The model under review builds one solid part; all positions refer to its coordinate system, in mm. A direction names the side the tool comes from. Round coordinates to 2 decimals unless told otherwise and drop trailing zeros. Order: outer loops, then holes, each group sorted by start corner. A loop starts at its lowest first (then second) coordinate and runs counter-clockwise, first axis right, second up. Notation, with made-up numbers: M 46.5,-16.5 L 102.5,-16.5 A25 cw 102.5,4.5 Z; hole C -39,36.5 d5. An arc over 180 degrees is marked long. Answer as a JSON object with one key per item and string values. Group by question number.
1) Consider section C-C, the plane x = 13. Write out the cut boundary in (y, z), then the cut area to 3 significant figures.
2) Insertion check: pin 1 Ø2 at (x, z) = (18.5, 14.5) entering from -Y; pin 2 Ø10 at (x, z) = (-16, 21) entering from +Y. Each pin has a flat end and moves straight along its axis. Give the tip position at first contact, or say it passes through.
3) Consider section A-A, the plane z = 0. Write out the cut boundary in (x, y), then the cut area to 3 significant figures.
4) Consider section B-B, the plane x = 0. Write out the cut boundary in (y, z).
5) To check wall thickness, follow line 1 (X direction, y = 33.5, z = 0); line 2 (Y direction, x = 17, z = 8); line 3 (Y direction, x = -23, z = -7). State the ranges of each line that lie inside material, in increasing order.
6) Consider section D-D, the plane y = 32.75. Write out the cut boundary in (x, z), then the cut area to 3 significant figures.
7) For faces 1 (the cylindrical face through (20.013, 37.121, 4.444)), 2 (the cylindrical face through (0, 35, 22)), 3 (the flat face through (0, 34.1, -5)), list the 3-axis set-ups (+Z, -Z, +X, -X, +Y, -Y) from which the entire face can be reached by the end or side of a thin tool; tool diameter is ignored.
8) The part is to be moulded in two halves that separate along Z. For faces 4 (the flat face through (14, 35.6, -16)), 5 (the cylindrical face through (7.46, 34.84, -22.37)), 6 (the cylindrical face through (-26.274, 33.135, 3.45)), say which applies: +Z half, -Z half, draft (parallel to the pull), parting line (faces both ways), or undercut.
```python
from build123d import *

# Parameters (mm, degrees)
SKETCH_3_W          = 2.645592797
SKETCH_3_H          = 5.492550126
CUT_EXTRUDE_START   = -20
CUT_EXTRUDE_2_DEPTH = 20
CUT_EXTRUDE_START_2 = -10
CUT_EXTRUDE_1_DEPTH = 10


with BuildPart() as part:
    # Эскиз1 → Повернуть1 (revolve)
    with BuildSketch(Plane.XY, mode=Mode.PRIVATE) as revolve_1_sk:
        Polygon((-26.5, 30.6), (-26.5, 35.6), (-20.5, 35.6), (-20.5, 38.6), (-1.75, 38.6), (-1.75, 34.1), (-24.523884272, 34.1), (-25, 34.1), (-25, 30.6), align=None)
    revolve(revolve_1_sk.sketch.rotate(Axis((0, 29.900525332, 0), (0, 1, 0)), 270), axis=Axis((0, 29.900525332, 0), (0, 1, 0)))

    # Эскиз3 → Вырез-Повернуть1 (revolve, cut)
    with BuildSketch(Plane.XY, mode=Mode.PRIVATE) as cut_revolve_1_sk:
        with Locations((11.677203602, 35.853724937)):
            Rectangle(SKETCH_3_W, SKETCH_3_H)
    revolve(cut_revolve_1_sk.sketch.rotate(Axis((13, 30.6, 0), (0, 1, 0)), 180), axis=Axis((13, 30.6, 0), (0, 1, 0)), mode=Mode.SUBTRACT)

    # Эскиз5 → Вырез-Вытянуть2 (cut)
    with BuildSketch(Plane(origin=(0, 35.6, 0), x_dir=(1, 0, 0), z_dir=(0, 1, 0)).offset(CUT_EXTRUDE_START)):
        with BuildLine():
            ThreePointArc((-5.617021277, -21.270850288), (-7.450285247, -22.338156812), (-6.382978723, -24.171420782))
            ThreePointArc((-6.382978723, -24.171420782), (0, -25), (6.382978723, -24.171420782))
            ThreePointArc((6.382978723, -24.171420782), (7.450285247, -22.338156812), (5.617021277, -21.270850288))
            ThreePointArc((5.617021277, -21.270850288), (0, -22), (-5.617021277, -21.270850288))
        make_face()
        with BuildLine():
            ThreePointArc((6.382978723, 24.171420782), (7.450285247, 22.338156812), (5.617021277, 21.270850288))
            ThreePointArc((5.617021277, 21.270850288), (0, 22), (-5.617021277, 21.270850288))
            ThreePointArc((-5.617021277, 21.270850288), (-7.450285247, 22.338156812), (-6.382978723, 24.171420782))
            ThreePointArc((-6.382978723, 24.171420782), (0, 25), (6.382978723, 24.171420782))
        make_face()
    extrude(amount=CUT_EXTRUDE_2_DEPTH, mode=Mode.SUBTRACT)

    # Эскиз4 → Вырез-Вытянуть1 (cut)
    with BuildSketch(Plane(origin=(0, 35.6, 0), x_dir=(1, 0, 0), z_dir=(0, 1, 0)).offset(CUT_EXTRUDE_START_2)):
        with BuildLine():
            ThreePointArc((-5.617021277, -21.270850288), (0, -22), (5.617021277, -21.270850288))
            ThreePointArc((5.617021277, -21.270850288), (7.450285247, -22.338156812), (6.382978723, -24.171420782))
            ThreePointArc((6.382978723, -24.171420782), (0, -25), (-6.382978723, -24.171420782))
            ThreePointArc((-6.382978723, -24.171420782), (-7.450285247, -22.338156812), (-5.617021277, -21.270850288))
        make_face()
        with BuildLine():
            ThreePointArc((6.382978723, 24.171420782), (7.450285247, 22.338156812), (5.617021277, 21.270850288))
            ThreePointArc((5.617021277, 21.270850288), (0, 22), (-5.617021277, 21.270850288))
            ThreePointArc((-5.617021277, 21.270850288), (-7.450285247, 22.338156812), (-6.382978723, 24.171420782))
            ThreePointArc((-6.382978723, 24.171420782), (0, 25), (6.382978723, 24.171420782))
        make_face()
    extrude(amount=CUT_EXTRUDE_1_DEPTH, mode=Mode.SUBTRACT)


solid = part.part
```
Results list:
{
 "1": {"outline": "M 30.6,-23.09 L 35.6,-23.09 L 35.6,-15.85 L 38.6,-15.85 L 38.6,-2.65 L 34.1,-2.65 L 34.1,-21.35 L 30.6,-21.35 Z; M 30.6,21.35 L 34.1,21.35 L 34.1,2.65 L 38.6,2.65 L 38.6,15.85 L 35.6,15.85 L 35.6,23.09 L 30.6,23.09 Z", "area": "153 mm^2"},
 "2": {"pin 1": "y = 34.1", "pin 2": "y = 35.6"},
 "3": {"outline": "M -26.5,30.6 L -25,30.6 L -25,34.1 L -1.75,34.1 L -1.75,38.6 L -20.5,38.6 L -20.5,35.6 L -26.5,35.6 Z; M 1.75,34.1 L 10.35,34.1 L 10.35,38.6 L 1.75,38.6 Z; M 15.65,34.1 L 25,34.1 L 25,30.6 L 26.5,30.6 L 26.5,35.6 L 20.5,35.6 L 20.5,38.6 L 15.65,38.6 Z", "area": "173 mm^2"},
 "4": {"outline": "M 30.6,-26.5 L 35.6,-26.5 L 35.6,-25 L 30.6,-25 Z; M 30.6,25 L 35.6,25 L 35.6,26.5 L 30.6,26.5 Z; M 34.1,-22 L 35.6,-22 L 35.6,-20.5 L 38.6,-20.5 L 38.6,-1.75 L 34.1,-1.75 Z; M 34.1,1.75 L 38.6,1.75 L 38.6,20.5 L 35.6,20.5 L 35.6,22 L 34.1,22 Z"},
 "5": {"line 1": "-26.5 to -25, 25 to 26.5", "line 2": "34.1 to 38.6", "line 3": "34.1 to 35.6"},
 "6": {"outline": "C 0,0 d53; hole C 0,0 d50", "area": "243 mm^2"},
 "7": {"face 1": "+Y", "face 2": "+Y, -Y", "face 3": "-Y"},
 "8": {"face 4": "draft", "face 5": "undercut", "face 6": "parting line"}
}
